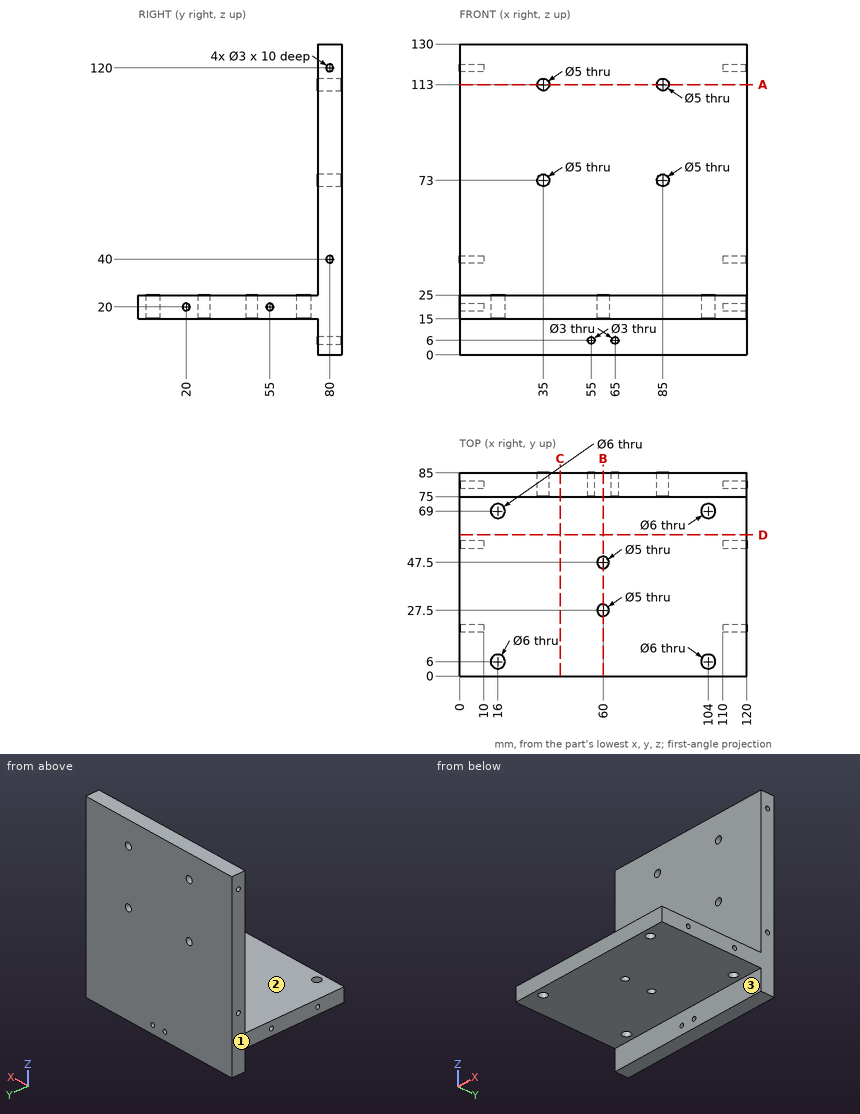
Input: dimensioned drawing with shaded views. Units: mm. Origin: part minimum x, y, z. A direction names the side the tool comes from. Coordinates: 2 decimals unless noted, no trailing zeros. Loops run counter-clockwise (first coordinate to the right, second up) from the corner with the lowest first, then second, coordinate; pieces in that order, holes last. Notation, with made-up numbers: M 67,43.5 L 106,43.5 A20 cw 106,70.5 Z; hole C 44,11 d5. An arc over 180 degrees is marked long. Put each result on its own line as item: value.
(1) Cut plane B-B on x = 60. Return the cut outline in (y, z), then the cut area to 3 significant figures.
Answer sheet:
outline: M 0,15 L 25,15 L 25,25 L 0,25 Z; M 30,15 L 45,15 L 45,25 L 30,25 Z; M 50,15 L 75,15 L 75,0 L 85,0 L 85,130 L 75,130 L 75,25 L 50,25 Z
area: 1,950 mm^2
(2) Cut plane D-D on y = 59. Return the cut outline in (x, z), then the cut area to 3 significant figures.
Answer sheet:
outline: M 0,15 L 120,15 L 120,25 L 0,25 Z
area: 1,200 mm^2
(3) First-contact query: pin 1 (4 mm diameter, centred on y = 55, z = 20, fed in from +X); pin 2 (1.8 mm diameter, centred on y = 20, z = 20, fed in from +X); pin 3 (10 mm diameter, centred on x = 102.5, y = 57.5, fed in from -Z); pin 4 (8 mm diameter, centred on x = 102, y = 58.5, fed in from +Z). Flat tips, straight axial feed; report the tip coordinate or a pass-through.
Answer sheet:
pin 1: stops at x = 120
pin 2: stops at x = 110
pin 3: stops at z = 15
pin 4: stops at z = 25
(4) Cut plane C-C on x = 42. Return the cut outline in (y, z).
Answer sheet:
outline: M 0,15 L 75,15 L 75,0 L 85,0 L 85,130 L 75,130 L 75,25 L 0,25 Z
(5) Cut plane A-A on z = 113. Return the cut outline in (x, y), then the cut area to 3 significant figures.
Answer sheet:
outline: M 0,75 L 32.5,75 L 32.5,85 L 0,85 Z; M 37.5,75 L 82.5,75 L 82.5,85 L 37.5,85 Z; M 87.5,75 L 120,75 L 120,85 L 87.5,85 Z
area: 1,100 mm^2
(6) Material intervals for probe 1 along Z at (x, y) = (115, 80); probe 2 along Z at (x, y) = (85, 81); probe 3 along X at (y, z) = (79, 113), sorted ascending.
Answer sheet:
probe 1: z = 0 to 38.5, 41.5 to 118.5, 121.5 to 130
probe 2: z = 0 to 70.5, 75.5 to 110.5, 115.5 to 130
probe 3: x = 0 to 32.5, 37.5 to 82.5, 87.5 to 120
(7) Access query for the marked faces 1, 2 and 3. Directions: +Z, -Z, +X, -X, +Y, -Y. A direction counts if a zero-diameter tool reaches every point of the face in a straight line with its end or side. Return the directions, or none.
Answer sheet:
face 1: +Z, -Z, -X, +Y, -Y
face 2: +Z, +X, -X, -Y
face 3: -Z, +X, -X, -Y
